```python
from build123d import *

# Parameters (mm, degrees)
SKETCH1_R           = 3.96875
SKETCH1_R_2         = 7.9375
SKETCH1_R_3         = 3.175
BOSS_EXTRUDE1_DEPTH = 6.35


with BuildPart() as part:
    # Sketch1 → Boss-Extrude1 (new body)
    with BuildSketch(Plane(origin=(0, 0, 0), x_dir=(1, 0, 0), z_dir=(0, 1, 0))):
        with BuildLine():
            Line((1.0715625, -14.247259739), (64.214375, -9.498173159))
            ThreePointArc((64.214375, -9.498173159), (72.11528772, -4.062319842), (71.282469536, 5.491702188))
            Line((71.282469536, 5.491702188), (36.357469536, 54.985054015))
            ThreePointArc((36.357469536, 54.985054015), (28.539380338, 59.018285224), (20.751674914, 54.926694223))
            Line((20.751674914, 54.926694223), (-11.734987629, 8.150013595))
            ThreePointArc((-11.734987629, 8.150013595), (-12.403089215, -7.091969697), (1.0715625, -14.247259739))
        make_face()
        with Locations(Location((28.575, 49.493351826, 0), (0, 0, 270))):
            Circle(SKETCH1_R, mode=Mode.SUBTRACT)
        with Locations(Location((0, 0, 0), (0, 0, 270))):
            Circle(SKETCH1_R_2, mode=Mode.SUBTRACT)
        with Locations(Location((63.5, 0, 0), (0, 0, 270))):
            Circle(SKETCH1_R, mode=Mode.SUBTRACT)
        with Locations(Location((14.2875, 24.746675913, 0), (0, 0, 270))):
            Circle(SKETCH1_R_3, mode=Mode.SUBTRACT)
        with Locations(Location((31.75, 0, 0), (0, 0, 270))):
            Circle(SKETCH1_R_3, mode=Mode.SUBTRACT)
        with Locations(Location((45.471967279, 25.5481107, 0), (0, 0, 270))):
            Circle(SKETCH1_R_3, mode=Mode.SUBTRACT)
    extrude(amount=BOSS_EXTRUDE1_DEPTH)


solid = part.part
```
Geometry check sheet. Reference: the model listing, model coordinates, mm. Round coordinates to 2 decimals unless told otherwise and drop trailing zeros. Order: outer loops, then holes, each group sorted by start corner. A loop starts at its lowest first (then second) coordinate and runs counter-clockwise, first axis right, second up. Notation, with made-up numbers: (67.5, 59.5) -> (98.5, 59.5) arc R30 cw to (98.5, 96.5) -> close; hole circle Ø10 at (-26.75, 88). An arc over 180 degrees is marked (long way). Return JSON: item names as keys, results as strings. Group by question number.
Q1. Section check A-A, the plane z = 0. Count the separate pieces of the cut face and the enclosed holes in it, plus the area to 3 significant figures.
Q2. Gauge pin test, flat ends, axial feed: pin 1 (10 mm diameter, centred on x = 14.29, z = -24.75, fed in from -Y); pin 2 (1 mm diameter, centred on y = 3, z = -3, fed in from +X); pin 3 (5 mm diameter, centred on x = 31.75, z = 0, fed in from +Y); pin 4 (1 mm diameter, centred on y = 5, z = -46.5, fed in from -X). Record the tip position at first contact, or that the pin passes through.
Q3. Section check D-D, the plane z = -15. Record the boundary of the cut face in (x, y), plus the area to 3 significant figures.
Q4. Release check for a two-part mould opening along X. For faces 1 (the cylindrical face through (28.65, 3.13, -0.69)), 2 (the flat face through (54.064, 3.131, -29.892)), 3 (the cylindrical face through (28.667, 3.131, -59.018)) record: released by +X, released by -X, zero draft, split by the parting line, or undercut.
Q5. Section check B-B, the plane x = 0. Record the boundary of the cut face in (y, z), plus the area to 3 significant figures.
Q6. Material ranges on probe 1 along X at (y, z) = (4, 0) (1 decimal); probe 2 along X at (y, z) = (3, -26); probe 3 along X at (y, z) = (3, 2.5), recorded low to high. Write a range as from..to.
Numbers:
{
 "1": {"separate pieces": "4", "enclosed holes": "0", "area": "363 mm^2"},
 "2": {"pin 1": "y = 0", "pin 2": "x = 72.69", "pin 3": "through", "pin 4": "x = 14.55"},
 "3": {"outline": "(-6.98, 0) -> (64.57, 0) -> (64.57, 6.35) -> (-6.98, 6.35) -> close", "area": "454 mm^2"},
 "4": {"face 1": "undercut", "face 2": "released by +X", "face 3": "split by the parting line"},
 "5": {"outline": "(0, -25.05) -> (6.35, -25.05) -> (6.35, -7.94) -> (0, -7.94) -> close; (0, 7.94) -> (6.35, 7.94) -> (6.35, 14.29) -> (0, 14.29) -> close", "area": "149 mm^2"},
 "6": {"probe 1": "-14.3..-7.9, 7.9..28.6, 34.9..59.5, 67.5..73", "probe 2": "0.66..11.37, 17.2..42.33, 48.61..56.81", "probe 3": "-14.07..-7.53, 7.53..29.79, 33.71..60.42, 66.58..72.69"}
}
